from build123d import *

# Parameters (mm, degrees)
F0_W      = 20
F0_H      = 20
F1_DEPTH  = 20
F2_W      = 11
F2_H      = 11
F3_DEPTH  = 25
F4_W      = 6
F4_H      = 6
F5_DEPTH  = 26
F6_W      = 23.7
F6_H      = 6
F7_DEPTH  = 0.1
F8_W      = 0.44082
F8_H      = 6
F9_DEPTH  = 40
F10_R     = 5
F11_DEPTH = 10


with BuildPart() as f1:
    # F0 (on Front) → F1 (new body)
    with BuildSketch(Plane.XZ):
        Rectangle(F0_W, F0_H)
    extrude(amount=F1_DEPTH)

    # F2 (on face) → F3 (cut)
    with BuildSketch(Plane.XY.offset(10)):
        with Locations((0, -10)):
            Rectangle(F2_W, F2_H)
    extrude(amount=-F3_DEPTH, mode=Mode.SUBTRACT)

    # F4 (on face) → F5 (join)
    with BuildSketch(Plane.XZ.offset(20)):
        Rectangle(F4_W, F4_H)
    extrude(amount=F5_DEPTH)

    # F6 (on face) → F7 (join)
    with BuildSketch(Plane.XZ.offset(46)):
        Rectangle(F6_W, F6_H)
    extrude(amount=F7_DEPTH)

    # F8 (on face) → F9 (join)
    with BuildSketch(Plane.XZ.offset(46.1)):
        with Locations((-11.62959, 0)):
            Rectangle(F8_W, F8_H)
        with Locations((11.62959, 0)):
            Rectangle(F8_W, F8_H)
    extrude(amount=F9_DEPTH)

    # F10 (on face) → F11 (cut)
    with BuildSketch(Plane(origin=(0, 0, 0), x_dir=(-1, 0, 0), z_dir=(0, 1, 0))):
        Circle(F10_R)
    extrude(amount=-F11_DEPTH, mode=Mode.SUBTRACT)


solid = f1.part
Source: CAD feature listing. Evaluate the final solid. Frame: model axes, mm. A direction names the side the tool comes from. Coordinates: 2 decimals unless noted, no trailing zeros. Order: outer loops, then holes, each group sorted by start corner. A loop starts at its lowest first (then second) coordinate and runs counter-clockwise, first axis right, second up.
Item 1: Pull-direction query (Y, two-part tool) for faces 4 (the face through (0, -3, 10)), 5 (the face through (0, -46.1, 0)), 6 (the face through (-3, -33, 0)); classes: pulls with the +Y half, pulls with the -Y half, needs draft (parallel to the pull), parting line crosses it, or undercut.
Output values:
face 4: needs draft
face 5: pulls with the -Y half
face 6: undercut
Item 2: Cut plane A-A (y = -62). Return loops of the section in (x, z), plus the area to 3 significant figures.
Output values:
outline: (-11.85, -3) - (-11.41, -3) - (-11.41, 3) - (-11.85, 3) - close; (11.41, -3) - (11.85, -3) - (11.85, 3) - (11.41, 3) - close
area: 5.29 mm2
Item 3: Cut plane B-B (x = 0). Return loops of the section in (y, z).
Output values:
outline: (-46.1, -3) - (-20, -3) - (-20, -10) - (-15.5, -10) - (-15.5, 10) - (-20, 10) - (-20, 3) - (-46.1, 3) - close; (-4.5, -10) - (0, -10) - (0, -5) - (-4.5, -5) - close; (-4.5, 5) - (0, 5) - (0, 10) - (-4.5, 10) - close
Item 4: Cut plane D-D (x = 3.75). Return loops of the section in (y, z), plus the area to 3 significant figures.
Output values:
outline: (-46.1, -3) - (-46, -3) - (-46, 3) - (-46.1, 3) - close; (-20, -10) - (-15.5, -10) - (-15.5, 10) - (-20, 10) - close; (-4.5, -10) - (0, -10) - (0, -3.31) - (-4.5, -3.31) - close; (-4.5, 3.31) - (0, 3.31) - (0, 10) - (-4.5, 10) - close
area: 151 mm2
Item 5: Cut plane C-C (z = -7.25). Return loops of the section in (x, y).
Output values:
outline: (-10, -20) - (10, -20) - (10, 0) - (-10, 0) - close; hole (-5.5, -15.5) - (5.5, -15.5) - (5.5, -4.5) - (-5.5, -4.5) - close
Item 6: Set-up query: faces 1 (the face through (-2.7, -38.2, 3)), 2 (the face through (3, -33, 0)), 3 (the face through (5.5, -10, 0)). Return all of +Z, -Z, +X, -X, +Y, -Y with unobstructed straight access to the full face (end or side cutting, diameter ignored); none if empty.
Output values:
face 1: +Z, +X, -X, -Y
face 2: +Z, -Z, +X
face 3: +Z, -Z
Item 7: First-contact query: P1, Ø6, axis at x = 1, z = 3, coming from the -Y side; P2, Ø6, axis at y = -7.5, z = 4.5, coming from the -X side; P3, Ø1.8, axis at y = -39.5, z = 0.5, coming from the -X side; P4, Ø1, axis at y = -36.5, z = 4.5, coming from the -X side. Flat tips, straight axial feed; report the tip coordinate or a pass-through.
Output values:
P1: stops at y = -46.1
P2: stops at x = -10
P3: stops at x = -3
P4: passes through
Item 8: Material intervals for line 1 (Z direction, x = 0, y = -2.55); line 2 (Y direction, x = 2, z = 9); line 3 (X direction, y = -10, z = 3.5), sorted ascending.
Output values:
line 1: z = -10 to -5, 5 to 10
line 2: y = -20 to -15.5, -4.5 to 0
line 3: x = -10 to -5.5, 5.5 to 10
